```python
from build123d import *

# Parameters (mm, degrees)
BOX_W           = 150
BOX_H           = 200
BOX_DEPTH       = 150
SKETCH_W        = 179.911882
SKETCH_H        = 115.378512
SKETCH_W_2      = 179.911881
SKETCH_H_2      = 12.61254
POCKET_DEPTH    = 140
SKETCH001_R     = 40
SKETCH001_W     = 594.158722
SKETCH001_H     = 187.959229
SKETCH001_W_2   = 106.580839
SKETCH001_H_2   = 20.811958
POCKET001_DEPTH = 20
SKETCH002_R     = 6
POCKET002_DEPTH = 20


with BuildPart() as part:
    # Box → Box (new body)
    with BuildSketch(Plane.XY):
        with Locations((75, 100)):
            Rectangle(BOX_W, BOX_H)
    extrude(amount=BOX_DEPTH)

    # Sketch → Pocket (cut)
    with BuildSketch(Plane(origin=(0, 0, 0), x_dir=(0, -1, 0), z_dir=(-1, 0, 0))):
        with Locations((-99.900999, 79.694251)):
            Rectangle(SKETCH_W, SKETCH_H)
        with Locations((-99.925957, 9.698538)):
            Rectangle(SKETCH_W_2, SKETCH_H_2)
    extrude(amount=-POCKET_DEPTH, mode=Mode.SUBTRACT)

    # Sketch001 → Pocket001 (cut)
    with BuildSketch(Plane.XZ):
        with Locations((72.839142, 69.31189)):
            Circle(SKETCH001_R)
        with Locations((757.154067, 877.348939)):
            Rectangle(SKETCH001_W, SKETCH001_H)
        with Locations((72.430153, 125.12305)):
            Rectangle(SKETCH001_W_2, SKETCH001_H_2)
    extrude(amount=-POCKET001_DEPTH, mode=Mode.SUBTRACT)

    # Sketch002 → Pocket002 (cut)
    with BuildSketch(Plane.YZ.offset(150)):
        with Locations((116.542318, 42.688718)):
            Circle(SKETCH002_R)
        with Locations((136.542318, 42.688718)):
            Circle(SKETCH002_R)
    extrude(amount=-POCKET002_DEPTH, mode=Mode.SUBTRACT)


solid = part.part
```
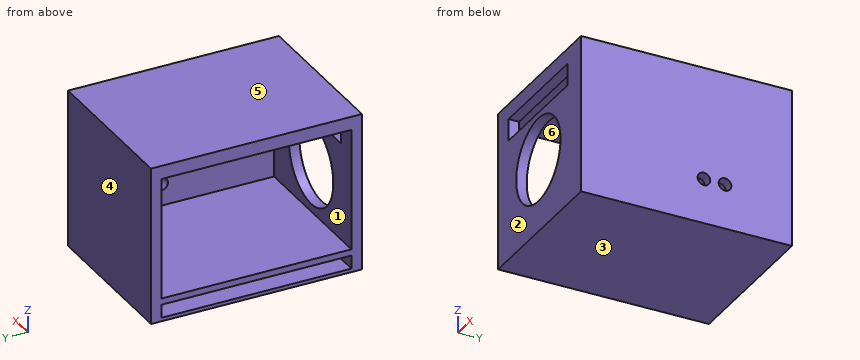
Work out the finished part from the listing and answer in its coordinate system (mm). Face numbers are marked on the shaded views. A direction names the side the tool comes from. Coordinates: 2 decimals unless noted, no trailing zeros. Loops run counter-clockwise (first coordinate to the right, second up) from the corner with the lowest first, then second, coordinate; pieces in that order, holes last. Notation, with made-up numbers: (60.5, 60.25) -> (104.5, 60.25) arc R26 ccw to (104.5, 84.25) -> close; hole circle Ø3 at (-10, 81). An arc over 180 degrees is marked (long way). Answer as CSV lines item,"result".
Q1. For a pull along Z with two mould halves and no side action, classify the marked faces 3, 4, 5 and 6 as +Z half, -Z half, draft (parallel to the pull), parting line (faces both ways), or undercut.
Findings:
face 3,"-Z half"
face 4,"draft"
face 5,"+Z half"
face 6,"undercut"
Q2. The part is cut by section C-C on y = 66.5. Write down the section's boundary in (x, z) (1 decimal), and give its area (3 significant figures).
Findings:
outline,"(0, 0) -> (150, 0) -> (150, 150) -> (0, 150) -> (0, 137.4) -> (140, 137.4) -> (140, 22) -> (0, 22) -> (0, 16) -> (140, 16) -> (140, 3.4) -> (0, 3.4) -> close"
area,"4,580 mm²"
Q3. A tool of negligible diameter and unlimited length cuts with its end or side. For the marked faces 1 and 2, from which of +Z, -Z, +X, -X, +Y, -Y can it reach the whole face along a straight path? Write none if from no direction.
Findings:
face 1,"-X"
face 2,"+Z, -Z, +X, -X, -Y"
Q4. Each of these flat-tipped pins is pushed along its axis until it touches: pin 1 (6 mm diameter, centred on x = 68.5, y = 105, fed in from -Z); pin 2 (12 mm diameter, centred on y = 49.5, z = 66.5, fed in from -X). Where does it stop, or does it pass through?
Findings:
pin 1,"stops at z = 0"
pin 2,"stops at x = 140"
Q5. The part is cut by section B-B on x = 36. Write down the section's boundary in (y, z) (1 decimal), and give its area (3 significant figures).
Findings:
outline,"(0, 0) -> (200, 0) -> (200, 150) -> (0, 150) -> (0, 135.5) -> (9.9, 135.5) -> (9.9, 137.4) -> (189.9, 137.4) -> (189.9, 22) -> (9.9, 22) -> (9.9, 53.7) -> (0, 53.7) -> close; (0, 84.9) -> (9.9, 84.9) -> (9.9, 114.7) -> (0, 114.7) -> close; hole (10, 3.4) -> (189.9, 3.4) -> (189.9, 16) -> (10, 16) -> close"
area,"6,460 mm²"
Q6. The part is cut by section A-A on z = 131. Write down the section's boundary in (x, y).
Findings:
outline,"(0, 0) -> (19.14, 0) -> (19.14, 9.95) -> (0, 9.95) -> close; (0, 189.86) -> (140, 189.86) -> (140, 9.95) -> (125.72, 9.95) -> (125.72, 0) -> (150, 0) -> (150, 200) -> (0, 200) -> close"
Q7. The part is cut by section D-D on x = 64. Write down the section's boundary in (y, z) (1 decimal), and give its area (3 significant figures).
Findings:
outline,"(0, 0) -> (200, 0) -> (200, 150) -> (0, 150) -> (0, 135.5) -> (9.9, 135.5) -> (9.9, 137.4) -> (189.9, 137.4) -> (189.9, 22) -> (9.9, 22) -> (9.9, 30.3) -> (0, 30.3) -> close; (0, 108.3) -> (9.9, 108.3) -> (9.9, 114.7) -> (0, 114.7) -> close; hole (10, 3.4) -> (189.9, 3.4) -> (189.9, 16) -> (10, 16) -> close"
area,"5,990 mm²"
Q8. Find the intervals of material crossed by probe 1 along Z at (x, y) = (101, 57) (1 decimal); probe 2 along Y at (x, z) = (127, 58.5); probe 3 along Y at (x, z) = (60, 6.5), in increasing order.
Findings:
probe 1,"z = 0 to 3.4, 16 to 22, 137.4 to 150"
probe 2,"y = 0 to 9.95, 189.86 to 200"
probe 3,"y = 0 to 9.97, 189.88 to 200"
